The drawing under review shows one solid part. Ordinate dimensions are in mm from its lowest x, y, z. A direction names the side the tool comes from. Coordinates: 2 decimals unless noted, no trailing zeros. Order: outer loops, then holes, each group sorted by start corner. A loop starts at its lowest first (then second) coordinate and runs counter-clockwise, first axis right, second up. Notation, with made-up numbers: (-14, -36) - (35, -36) arc R4 cw to (35, -31) - close; hole circle Ø5 at (63.25, 3). An arc over 180 degrees is marked (long way). Write each question's results on one line, items separated by ' | '. Start each with the question number.
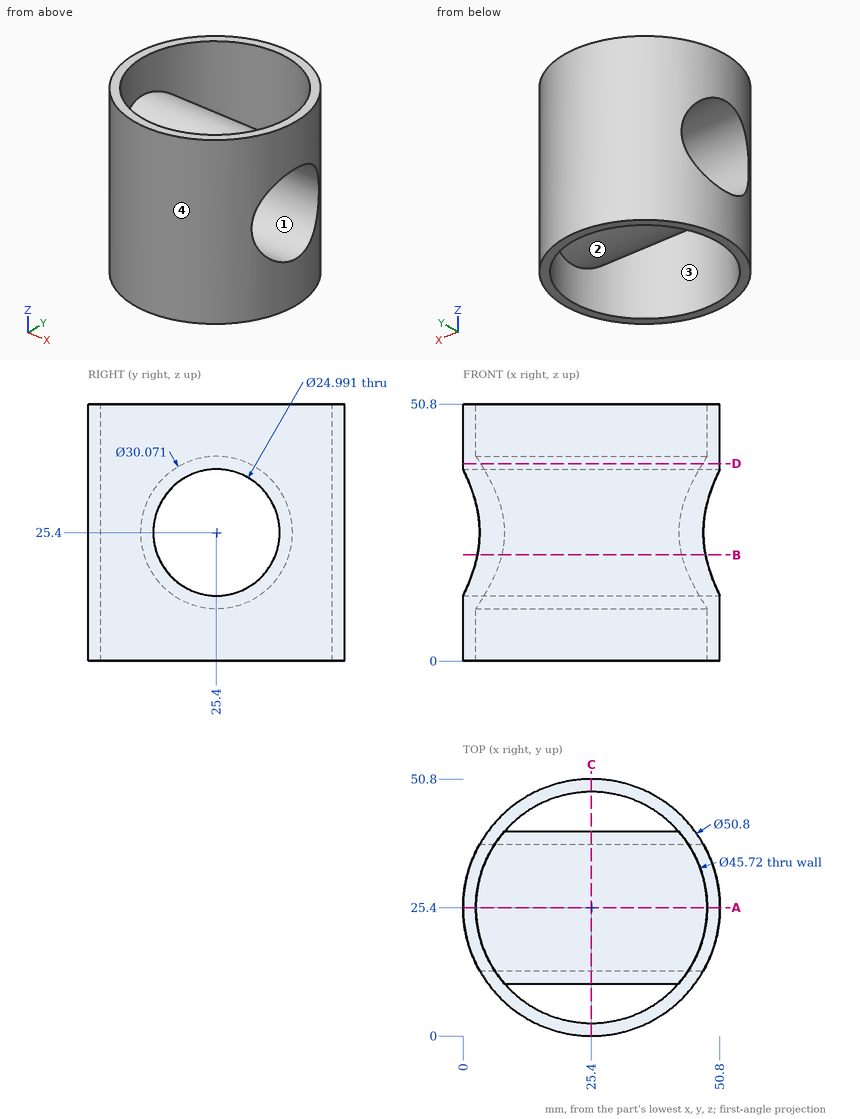
(1) Take a section at A-A (y = 25.4). State the section outline as (x, z) points, plus the area to 3 significant figures.
(2) Clearance check with flat-ended pins moving along their axes: pin 1 (8 mm diameter, centred on x = 28.5, z = 35, fed in from +Y); pin 2 (1 mm diameter, centred on x = 11, z = 32.5, fed in from -Y); pin 3 (3 mm diameter, centred on x = 42.5, y = 23, fed in from +Z); pin 4 (20 mm diameter, centred on y = 25.4, z = 25.4, fed in from +X). State where each tip first meets the part, or that it passes through.
(3) Tool access review of the marked faces 1 and 2: name each direction out of +Z, -Z, +X, -X, +Y, -Y from which nothing blocks a thin tool from reaching the whole face with its end or side.
(4) Take a section at D-D (z = 39). State the section outline as (x, y) points.
(5) To check wall thickness, follow line 1 along Z through (x, y) = (36.5, 25.5) (3 decimals); line 2 along Y through (x, z) = (26, 5.5); line 3 along Y through (x, z) = (38.5, 31). State the ranges of each line that lie inside material, in increasing order. Write a range as [from, to].
(6) Take a section at B-B (z = 21). State the section outline as (x, y) points.
(7) Mouldability with a two-part tool opening along Y and no side actions: class the marked faces 3 and 4 as +Y half, -Y half, draft (parallel to the pull), parting line (faces both ways), or undercut.
(8) Take a section at C-C (x = 25.4). State the section outline as (y, z) points.
Worked out:
1) outline: (0, 0) - (2.54, 0) - (2.54, 10.36) - (48.26, 10.36) - (48.26, 0) - (50.8, 0) - (50.8, 12.9) - (0, 12.9) - close; (0, 37.9) - (50.8, 37.9) - (50.8, 50.8) - (48.26, 50.8) - (48.26, 40.44) - (2.54, 40.44) - (2.54, 50.8) - (0, 50.8) - close | area: 363 mm^2
2) pin 1: y = 50.8 | pin 2: y = 4.14 | pin 3: z = 40.41 | pin 4: through
3) face 1: +X, -X | face 2: none
4) outline: circle Ø50.8 at (25.4, 25.4); hole (3.46, 18.99) arc R22.86 ccw to (47.34, 18.99) - close; hole (3.46, 31.81) - (47.34, 31.81) arc R22.86 ccw to start
5) line 1: [10.365, 12.905], [37.895, 40.435] | line 2: [0.01, 2.55], [48.25, 50.79] | line 3: [3.64, 6.67], [11.45, 14.23], [36.57, 39.35], [44.13, 47.16]
6) outline: (2.85, 13.7) arc R25.4 ccw to (47.95, 13.7) - close; (2.85, 37.1) - (47.95, 37.1) arc R25.4 ccw to start; hole (7.63, 11.02) arc R22.86 ccw to (43.17, 11.02) - close; hole (7.63, 39.78) - (43.17, 39.78) arc R22.86 ccw to start
7) face 3: undercut | face 4: parting line
8) outline: (0, 0) - (2.54, 0) - (2.54, 50.8) - (0, 50.8) - close; circle Ø30.07 at (25.4, 25.4); (48.26, 0) - (50.8, 0) - (50.8, 50.8) - (48.26, 50.8) - close; hole circle Ø24.99 at (25.4, 25.4)
